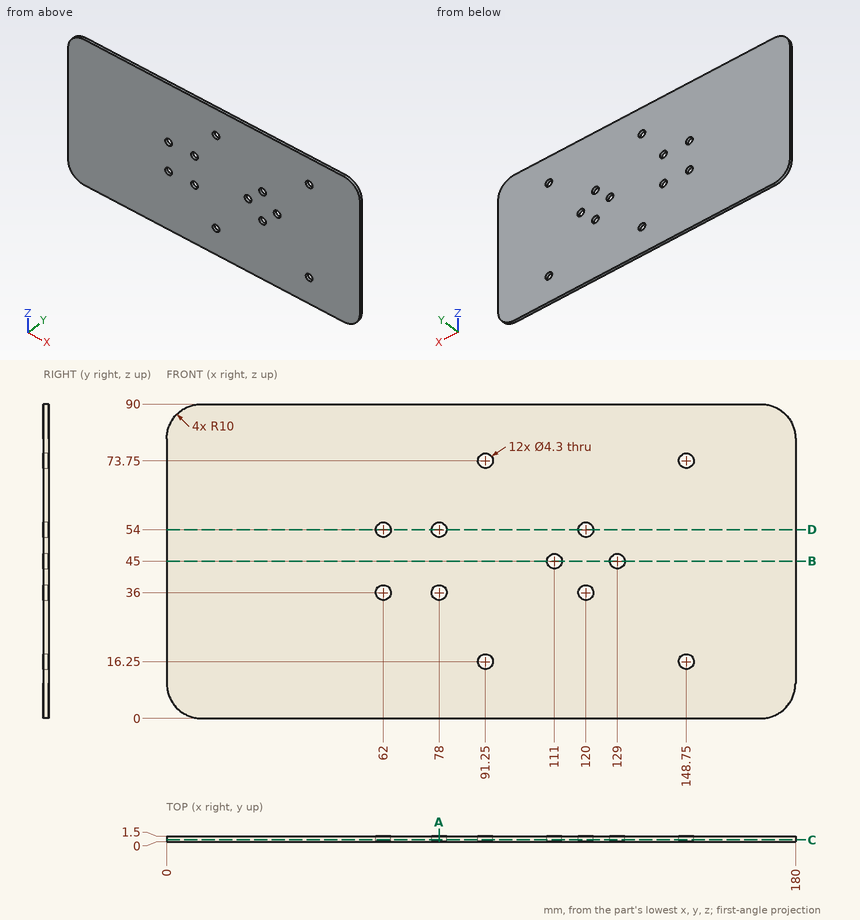
Could you check a few things on this drawing? It's one solid part, dimensions in mm from its lowest x, y, z. Coordinates: 2 decimals unless noted, no trailing zeros. Write each loop counter-clockwise with the first axis right and the second up, starting at its lowest first coordinate (ties: lowest second). Pieces come first, ordered by that corner, then holes. Notation, with made-up numbers: M 18,84 L 62,84 A21 cw 62,106 Z; hole C -15,62.5 d3. An arc over 180 degrees is marked long. Answer as CSV lines item,"result". Start each with the question number.
Q1. Suppose I cut it at A-A, the plane x = 78. List the corners of the cut face in (y, z) for me, then the cut area to 3 significant figures.
Q2. Will this pin go through, and if not, where does the flat tip stop? pin 1 Ø5.5 at (x, z) = (62, 54) entering from +Y.
Q3. Suppose I cut it at B-B, the plane z = 45. List the corners of the cut face in (x, y) for me, then the cut area to 3 significant figures.
Q4. Suppose I cut it at C-C, the plane y = 0.5. State how many separate pieces and enclosed holes the cut face has, then the cut area to 3 significant figures.
Q5. I need wall thicknesses on probe 1 along X at (y, z) = (0.3, 36); probe 2 along X at (y, z) = (0.75, 45); probe 3 along X at (y, z) = (0.7, 73.75). Which ranges of each line are inside material? Lowest first, please. Write a range as [from, to].
Q6. Suppose I cut it at D-D, the plane z = 54. List the corners of the cut face in (x, y) for me, then the cut area to 3 significant figures.
Entries:
1,outline,"M 0,0 L 1.5,0 L 1.5,33.85 L 0,33.85 Z; M 0,38.15 L 1.5,38.15 L 1.5,51.85 L 0,51.85 Z; M 0,56.15 L 1.5,56.15 L 1.5,90 L 0,90 Z"
1,area,"122 mm²"
2,pin 1,"stops at y = 1.5"
3,outline,"M 0,0 L 108.85,0 L 108.85,1.5 L 0,1.5 Z; M 113.15,0 L 126.85,0 L 126.85,1.5 L 113.15,1.5 Z; M 131.15,0 L 180,0 L 180,1.5 L 131.15,1.5 Z"
3,area,"257 mm²"
4,separate pieces,"1"
4,enclosed holes,"12"
4,area,"15,900 mm²"
5,probe 1,"x = [0, 59.85], [64.15, 75.85], [80.15, 117.85], [122.15, 180]"
5,probe 2,"x = [0, 108.85], [113.15, 126.85], [131.15, 180]"
5,probe 3,"x = [0, 89.1], [93.4, 146.6], [150.9, 180]"
6,outline,"M 0,0 L 59.85,0 L 59.85,1.5 L 0,1.5 Z; M 64.15,0 L 75.85,0 L 75.85,1.5 L 64.15,1.5 Z; M 80.15,0 L 117.85,0 L 117.85,1.5 L 80.15,1.5 Z; M 122.15,0 L 180,0 L 180,1.5 L 122.15,1.5 Z"
6,area,"251 mm²"
